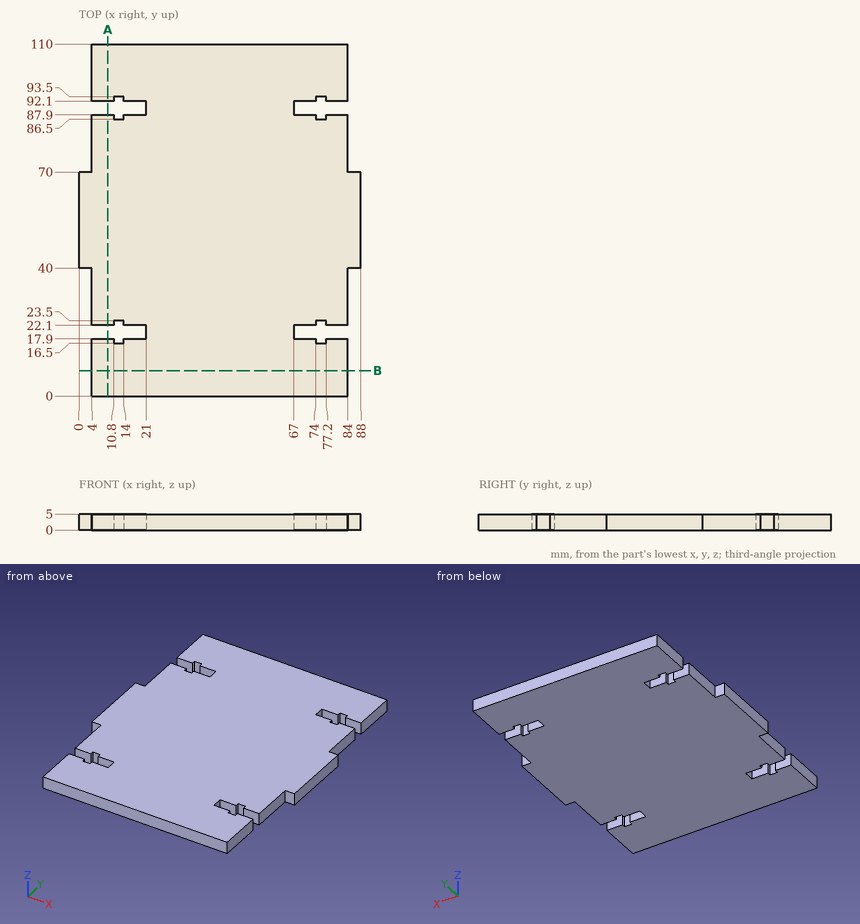
Geometry check sheet. Reference: drawing and pictorial views, mm from the part's lowest x, y, z. Round coordinates to 2 decimals unless told otherwise and drop trailing zeros. Loops run counter-clockwise (first coordinate to the right, second up) from the corner with the lowest first, then second, coordinate; pieces in that order, holes last. Notation, with made-up numbers: (-4, 18) - (53, 18) arc R30 ccw to (53, 49) - close; hole circle Ø10 at (8.5, 48.5). An arc over 180 degrees is marked (long way). Use a Markdown table: item, result.
Q1. Material ranges on line 1 (Y direction, x = 17.5, z = 2.85); line 2 (X direction, y = 87, z = 0.8); line 3 (X direction, y = 26, z = 2.2), recorded low to high.
Solutions:
| item | result |
|---|---|
| line 1 | y = 0 to 17.9, 22.1 to 87.9, 92.1 to 110 |
| line 2 | x = 4 to 10.8, 14 to 74, 77.2 to 84 |
| line 3 | x = 4 to 84 |
Q2. Go/stop test with flat-tipped pins: P1, Ø1.2, axis at x = 2, z = 3, coming from the +Y side; P2, Ø1.1, axis at y = 92.5, z = 3.5, coming from the -X side; P3, Ø2, axis at y = 89.5, z = 1.5, coming from the -X side. Record where each tip stops, or that it passes through.
Solutions:
| item | result |
|---|---|
| P1 | stops at y = 70 |
| P2 | stops at x = 4 |
| P3 | stops at x = 21 |
Q3. Cross-section at A-A on x = 9. Record the cut outline in (y, z), plus the area to 3 significant figures.
Solutions:
| item | result |
|---|---|
| outline | (0, 0) - (17.9, 0) - (17.9, 5) - (0, 5) - close; (22.1, 0) - (87.9, 0) - (87.9, 5) - (22.1, 5) - close; (92.1, 0) - (110, 0) - (110, 5) - (92.1, 5) - close |
| area | 508 mm2 |
Q4. Cross-section at B-B on y = 8. Record the cut outline in (x, z), plus the area to 3 significant figures.
Solutions:
| item | result |
|---|---|
| outline | (4, 0) - (84, 0) - (84, 5) - (4, 5) - close |
| area | 400 mm2 |
